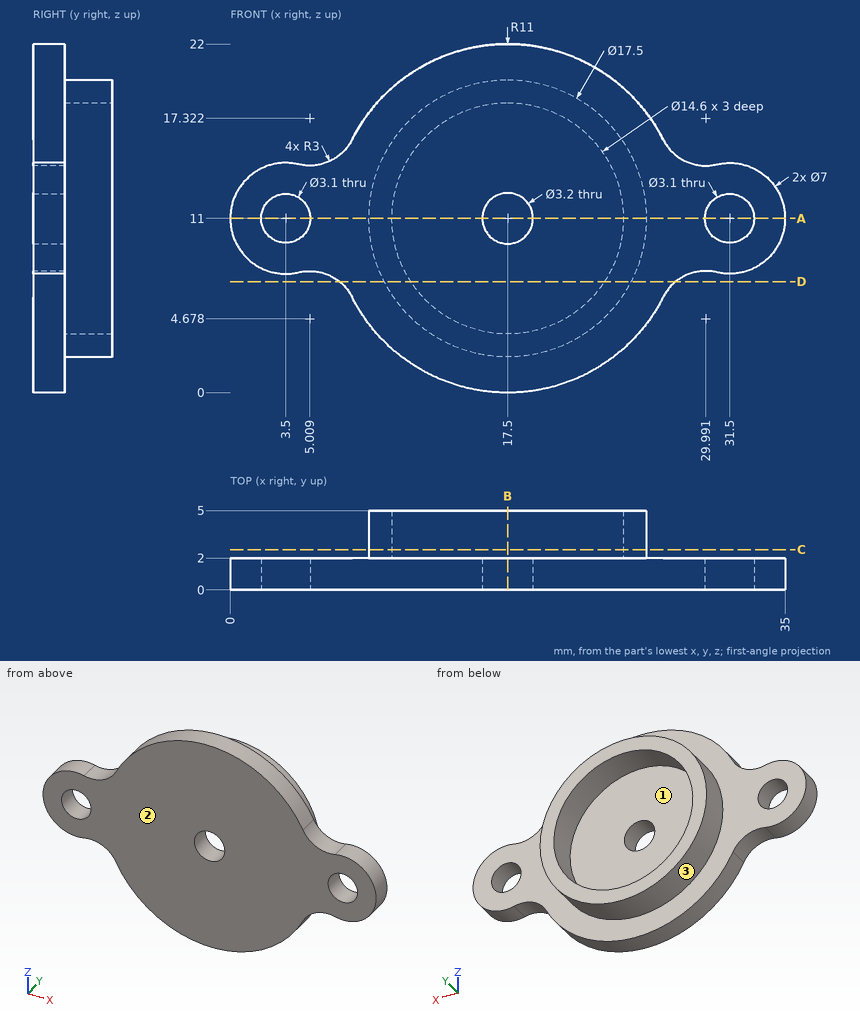
Verification items for this drawing (mm, ordinates from the low corner). Give positions to 0.01 mm unless a question says otherwise; leave off trailing zeros. Loops run counter-clockwise (first coordinate to the right, second up) from the corner with the lowest first, then second, coordinate; pieces in that order, holes last.
(1) Section check D-D on z = 7. Record the cut outline in (x, y).
From the geometry:
outline: (6.91, 0) - (28.09, 0) - (28.09, 2) - (25.28, 2) - (25.28, 5) - (23.61, 5) - (23.61, 2) - (11.39, 2) - (11.39, 5) - (9.72, 5) - (9.72, 2) - (6.91, 2) - close
(2) Section check B-B on x = 17.5. Record the cut outline in (y, z), then the cut area to 3 significant figures.
From the geometry:
outline: (0, 0) - (2, 0) - (2, 2.25) - (5, 2.25) - (5, 3.7) - (2, 3.7) - (2, 9.4) - (0, 9.4) - close; (0, 12.6) - (2, 12.6) - (2, 18.3) - (5, 18.3) - (5, 19.75) - (2, 19.75) - (2, 22) - (0, 22) - close
area: 46.3 mm2
(3) Thickness scan on L1, parallel to X at y = 0.55, z = 11; L2, parallel to X at y = 4.35, z = 11; L3, parallel to Z at x = 22.5, y = 3.9. Record the ranges inside material, lowest first.
From the geometry:
L1: x = 0 to 1.95, 5.05 to 15.9, 19.1 to 29.95, 33.05 to 35
L2: x = 8.75 to 10.2, 24.8 to 26.25
L3: z = 3.82 to 5.68, 16.32 to 18.18
(4) Depth check by flat-ended pin: pin 1 Ø3 at (x, z) = (31.5, 11) entering from +Y; pin 2 Ø2 at (y, z) = (3.5, 10) entering from -X; pin 3 Ø5 at (x, z) = (3.5, 11) entering from +Y; pin 4 Ø3 at (y, z) = (2.5, 14) entering from -X. Enter the tip coordinate at first touch or a pass-through.
From the geometry:
pin 1: passes through
pin 2: stops at x = 8.75
pin 3: stops at y = 2
pin 4: stops at x = 0.38
(5) Section check A-A on z = 11. Record the cut outline in (x, y).
From the geometry:
outline: (0, 0) - (1.95, 0) - (1.95, 2) - (0, 2) - close; (5.05, 0) - (15.9, 0) - (15.9, 2) - (10.2, 2) - (10.2, 5) - (8.75, 5) - (8.75, 2) - (5.05, 2) - close; (19.1, 0) - (29.95, 0) - (29.95, 2) - (26.25, 2) - (26.25, 5) - (24.8, 5) - (24.8, 2) - (19.1, 2) - close; (33.05, 0) - (35, 0) - (35, 2) - (33.05, 2) - close
(6) Release check for a two-part mould opening along X. For the marked faces 1, 2 and 3 record: released by +X, released by -X, zero draft, split by the parting line, or undercut.
From the geometry:
face 1: undercut
face 2: zero draft
face 3: split by the parting line
(7) Section check C-C on y = 2.55. Record the cut outline in (x, z).
From the geometry:
outline: circle Ø17.5 at (17.5, 11); hole circle Ø14.6 at (17.5, 11)
